Job drawing, mm, ordinate dimensions from the low corner. One solid piece. A direction names the side the tool comes from. Give positions to 0.01 mm unless a question says otherwise; leave off trailing zeros. Order: outer loops, then holes, each group sorted by start corner. A loop starts at its lowest first (then second) coordinate and runs counter-clockwise, first axis right, second up. Notation, with made-up numbers: M 8,72 L 38,72 A22 cw 38,83 Z; hole C 62.5,68 d2. An arc over 180 degrees is marked long. One line per question, with ' | ' between items.
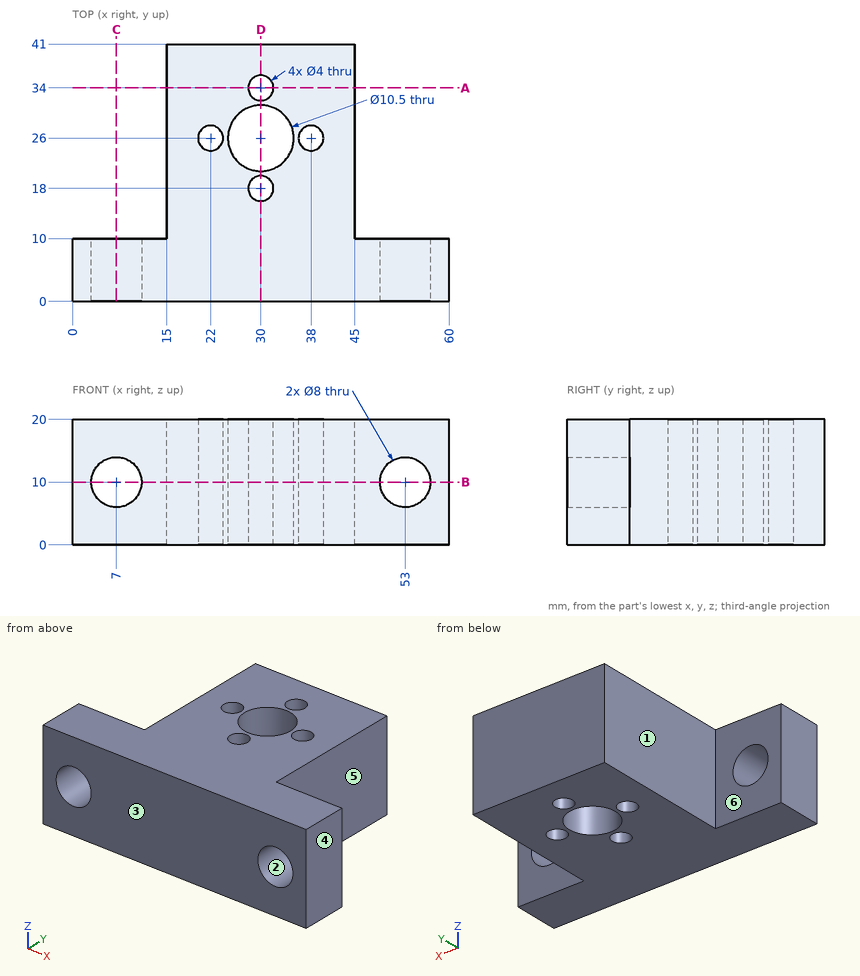
1. Slice it at C-C on x = 7. Give the cut face in (y, z).
Worked out:
outline: M 0,0 L 10,0 L 10,6 L 0,6 Z; M 0,14 L 10,14 L 10,20 L 0,20 Z
2. Slice it at D-D on x = 30. Give the cut face in (y, z).
Worked out:
outline: M 0,0 L 16,0 L 16,20 L 0,20 Z; M 20,0 L 20.75,0 L 20.75,20 L 20,20 Z; M 31.25,0 L 32,0 L 32,20 L 31.25,20 Z; M 36,0 L 41,0 L 41,20 L 36,20 Z
3. Slice it at B-B on z = 10. Give the cut face in (x, y), then the cut area to 3 significant figures.
Worked out:
outline: M 0,0 L 3,0 L 3,10 L 0,10 Z; M 11,0 L 49,0 L 49,10 L 45,10 L 45,41 L 15,41 L 15,10 L 11,10 Z; M 57,0 L 60,0 L 60,10 L 57,10 Z; hole C 22,26 d4; hole C 30,26 d10.5; hole C 30,18 d4; hole C 30,34 d4; hole C 38,26 d4 | area: 1,230 mm2
4. Tool access for the marked faces 4, 5 and 6: list every direction of +Z, -Z, +X, -X, +Y, -Y with a clear straight run to the whole face (end or side of a thin tool).
Worked out:
face 4: +Z, -Z, +X, +Y, -Y | face 5: +Z, -Z, +X, +Y | face 6: +Z, -Z, -X, +Y
5. Slice it at A-A on y = 34. Give the cut face in (x, z), then the cut area to 3 significant figures.
Worked out:
outline: M 15,0 L 28,0 L 28,20 L 15,20 Z; M 32,0 L 45,0 L 45,20 L 32,20 Z | area: 520 mm2
6. Probe L1, parallel to X at y = 6, z = 10.25; L2, parallel to Y at x = 30, z = 10.5; L3, parallel to Z at x = 7, y = 9. List the from-to ranges inside material, lowest first. Write a range as from..to.
Worked out:
L1: x = 0..3.01, 10.99..49.01, 56.99..60 | L2: y = 0..16, 20..20.75, 31.25..32, 36..41 | L3: z = 0..6, 14..20
7. Drop flat-ended pins along their axis: pin 1 (6 mm diameter, centred on y = 32, z = 5.5, fed in from +X); pin 2 (2.5 mm diameter, centred on x = 30, y = 34, fed in from +Z); pin 3 (10 mm diameter, centred on y = 22.5, z = 13, fed in from -X); pin 4 (3 mm diameter, centred on x = 6.5, z = 7, fed in from +Y). Give the stop position or say it passes through.
Worked out:
pin 1: stops at x = 45 | pin 2: passes through | pin 3: stops at x = 15 | pin 4: stops at y = 10
8. Mould opens along X. For the marked faces 1, 2 and 3 say: released by +X, released by -X, zero draft, split by the parting line, or undercut.
Worked out:
face 1: released by -X | face 2: undercut | face 3: zero draft
